```python
from build123d import *

# Parameters (mm, degrees)
BOSS_EXTRUDE1_DEPTH = 12.7
BOSS_EXTRUDE2_DEPTH = 11.43
BOSS_EXTRUDE3_DEPTH = 3.175
SKETCH25_W          = 101.6
SKETCH25_H          = 203.2
CUT_EXTRUDE16_DEPTH = 26.4
SKETCH31_W          = 40.64
SKETCH31_H          = 12.7
BOSS_EXTRUDE5_DEPTH = 3.175
SKETCH27_R          = 4.953
SKETCH27_R_2        = 12.7
SKETCH27_W          = 50.8
SKETCH27_H          = 50.8
CUT_EXTRUDE17_DEPTH = 0.0254
SKETCH28_W          = 23.8125
SKETCH28_H          = 11.509375
SKETCH28_W_2        = 11.509375
SKETCH28_H_2        = 23.8125
CUT_EXTRUDE18_DEPTH = 0.0254


with BuildPart() as part:
    # Sketch1 → Boss-Extrude1 (new body)
    with BuildSketch(Plane(origin=(0, 0, 0), x_dir=(1, 0, 0), z_dir=(0, 1, 0))):
        with BuildLine():
            Line((-31.75, 0), (31.75, 0))
            Line((31.75, 0), (31.75, 111.76))
            ThreePointArc((31.75, 111.76), (0, 122.90426271), (-31.75, 111.76))
            Line((-31.75, 111.76), (-31.75, 0))
        make_face()
    extrude(amount=BOSS_EXTRUDE1_DEPTH)

    # Sketch2 → Boss-Extrude2 (add)
    with BuildSketch(Plane.ZY.offset(31.75)):
        with BuildLine():
            Line((0, 0), (12.7, 0))
            ThreePointArc((12.7, 0), (21.680256121, 21.680256121), (0, 12.7))
            Line((0, 12.7), (0, 0))
        make_face()
    boss_extrude2 = extrude(amount=-BOSS_EXTRUDE2_DEPTH)

    # Mirror1: Boss-Extrude2 across plane
    add(boss_extrude2.mirror(Plane(origin=(0, 0, 0), x_dir=(0, 0, 1), z_dir=(1, 0, 0))))

    # Sketch24 → Boss-Extrude3 (add)
    with BuildSketch(Plane.XZ):
        with BuildLine():
            Line((20.32, 0), (-20.32, 0))
            Line((-20.32, 0), (-20.32, 12.7))
            Line((-20.32, 12.7), (-31.75, 12.7))
            Line((-31.75, 12.7), (-31.75, -111.76))
            ThreePointArc((-31.75, -111.76), (0, -122.90426271), (31.75, -111.76))
            Line((31.75, -111.76), (31.75, 12.7))
            Line((31.75, 12.7), (20.32, 12.7))
            Line((20.32, 12.7), (20.32, 0))
        make_face()
    extrude(amount=BOSS_EXTRUDE3_DEPTH)

    # Sketch25 → Cut-Extrude16 (cut, through all)
    with BuildSketch(Plane(origin=(0, 0, 0), x_dir=(-1, 0, 0), z_dir=(0, -1, 0))):
        with Locations((12.008205385, 70.319547201)):
            Rectangle(SKETCH25_W, SKETCH25_H)
    extrude(amount=-CUT_EXTRUDE16_DEPTH, mode=Mode.SUBTRACT)

    # Sketch31 → Boss-Extrude5 (add)
    with BuildSketch(Plane(origin=(0, 0, 0), x_dir=(1, 0, 0), z_dir=(0, 1, 0))):
        with Locations((0, -6.35)):
            Rectangle(SKETCH31_W, SKETCH31_H)
    extrude(amount=-BOSS_EXTRUDE5_DEPTH)

    # Sketch27 → Cut-Extrude17 (cut)
    with BuildSketch(Plane(origin=(0, 0, 0), x_dir=(1, 0, 0), z_dir=(0, 1, 0))):
        with Locations((19.05, 112.10926271)):
            Circle(SKETCH27_R)
        with Locations((-19.05, 112.10926271)):
            Circle(SKETCH27_R)
        with Locations((26.162, -6.25473729)):
            Circle(SKETCH27_R)
        with Locations((-26.162, -6.25473729)):
            Circle(SKETCH27_R)
        with Locations((0, 91.15426271)):
            Circle(SKETCH27_R_2)
        with Locations((0, 42.13226271)):
            Rectangle(SKETCH27_W, SKETCH27_H)
    extrude(amount=-CUT_EXTRUDE17_DEPTH, mode=Mode.SUBTRACT)

    # Sketch28 → Cut-Extrude18 (cut)
    with BuildSketch(Plane(origin=(0, 0, 0), x_dir=(1, 0, 0), z_dir=(0, 1, 0))):
        with Locations((-16.03375, 7.0088125)):
            Rectangle(SKETCH28_W, SKETCH28_H)
        with Locations((22.1853125, 85.12175)):
            Rectangle(SKETCH28_W_2, SKETCH28_H_2)
        with Locations((16.03375, 7.0088125)):
            Rectangle(SKETCH28_W, SKETCH28_H)
        with Locations((0, 113.33957521)):
            Rectangle(SKETCH28_W, SKETCH28_H)
        with Locations((-22.1853125, 85.12175)):
            Rectangle(SKETCH28_W_2, SKETCH28_H_2)
    extrude(amount=-CUT_EXTRUDE18_DEPTH, mode=Mode.SUBTRACT)


solid = part.part
```
Work out the finished part from the listing and answer in its coordinate system (mm). Give positions to 0.01 mm unless a question says otherwise; leave off trailing zeros. Loops run counter-clockwise (first coordinate to the right, second up) from the corner with the lowest first, then second, coordinate; pieces in that order, holes last. Notation, with made-up numbers: (15, 27) - (39, 27) arc R5 cw to (39, 36) - close; hole circle Ø8 at (4.5, 8). An arc over 180 degrees is marked (long way). Use CSV: the item, a comma, the result in double quotes. Start each with the question number.
(1) Find section B-B, the plane y = -2.5. Determine the outline of the cut face in (x, z).
(2) Each of these flat-tipped pins is pushed along its axis until it touches: pin 1 (1 mm diameter, centred on x = -6.5, z = -54.5, fed in from +Y); pin 2 (1 mm diameter, centred on x = 15.5, y = -2, fed in from -Z); pin 3 (1 mm diameter, centred on x = 15, y = -1, fed in from -Z). Where does it stop, or does it pass through?
(3) Find the intervals of material crossed by L1, parallel to Y at x = 7.5, z = -50 (3 decimals); L2, parallel to Z at x = -1, y = -1.1; L3, parallel to Z at x = -3, y = -2, in increasing order.
Results found:
1,outline,"(-31.75, -111.76) arc R50.8 ccw to (31.75, -111.76) - (31.75, 12.7) - (-31.75, 12.7) - close"
2,pin 1,"y = -0.03"
2,pin 2,"z = -120.64"
2,pin 3,"z = -120.79"
3,L1,"-3.175 to -0.025"
3,L2,"-122.89 to 12.7"
3,L3,"-122.82 to 12.7"
